```python
from build123d import *

# Parameters (mm, degrees)
SKETCH1_W           = 60
SKETCH1_H           = 28.5
BOSS_EXTRUDE1_DEPTH = 2
SKETCH2_W           = 60
SKETCH2_H           = 2
BOSS_EXTRUDE2_DEPTH = 35
SKETCH3_W           = 41
SKETCH3_H           = 28.5
BOSS_EXTRUDE3_DEPTH = 8
SKETCH4_W           = 20
SKETCH4_H           = 2
BOSS_EXTRUDE4_DEPTH = 20
SKETCH5_W           = 41
SKETCH5_H           = 22
CUT_EXTRUDE1_DEPTH  = 2
SKETCH6_R           = 1.5
CUT_EXTRUDE2_DEPTH  = 2
SKETCH7_R           = 1
BOSS_EXTRUDE5_DEPTH = 5
FILLET1_R           = 10
FILLET2_R           = 10
SKETCH8_R           = 1
CUT_EXTRUDE3_DEPTH  = 2


with BuildPart() as part:
    # Sketch1 → Boss-Extrude1 (new body)
    with BuildSketch(Plane(origin=(0, 0, 0), x_dir=(1, 0, 0), z_dir=(0, 1, 0))):
        Rectangle(SKETCH1_W, SKETCH1_H)
    extrude(amount=BOSS_EXTRUDE1_DEPTH)

    # Sketch2 → Boss-Extrude2 (add)
    with BuildSketch(Plane(origin=(0, 2, 0), x_dir=(1, 0, 0), z_dir=(0, 1, 0))):
        with Locations((0, 13.25)):
            Rectangle(SKETCH2_W, SKETCH2_H)
    extrude(amount=BOSS_EXTRUDE2_DEPTH)

    # Sketch3 → Boss-Extrude3 (add)
    with BuildSketch(Plane(origin=(0, 2, 0), x_dir=(1, 0, 0), z_dir=(0, 1, 0))):
        Rectangle(SKETCH3_W, SKETCH3_H)
    extrude(amount=BOSS_EXTRUDE3_DEPTH)

    # Sketch4 → Boss-Extrude4 (add)
    with BuildSketch(Plane(origin=(0, 10, 0), x_dir=(1, 0, 0), z_dir=(0, 1, 0))):
        with Locations((10.5, -13.25)):
            Rectangle(SKETCH4_W, SKETCH4_H)
    extrude(amount=BOSS_EXTRUDE4_DEPTH)

    # Sketch5 → Cut-Extrude1 (cut)
    with BuildSketch(Plane(origin=(0, 0, -14.25), x_dir=(-1, 0, 0), z_dir=(0, 0, -1))):
        with Locations((0, 21)):
            Rectangle(SKETCH5_W, SKETCH5_H)
    extrude(amount=-CUT_EXTRUDE1_DEPTH, mode=Mode.SUBTRACT)

    # Sketch6 → Cut-Extrude2 (cut)
    with BuildSketch(Plane(origin=(0, 0, -14.25), x_dir=(-1, 0, 0), z_dir=(0, 0, -1))):
        with Locations((-24, 25)):
            Circle(SKETCH6_R)
        with Locations((-24, 15)):
            Circle(SKETCH6_R)
    cut_extrude2 = extrude(amount=-CUT_EXTRUDE2_DEPTH, mode=Mode.SUBTRACT)

    # Mirror1: Cut-Extrude2 across plane
    add(cut_extrude2.mirror(Plane(origin=(0, 0, 0), x_dir=(0, 0, 1), z_dir=(1, 0, 0))), mode=Mode.SUBTRACT)

    # Sketch7 → Boss-Extrude5 (add)
    with BuildSketch(Plane.XY.offset(14.25)):
        with Locations(Location((10.5, 20, 0), (0, 0, 180))):
            Circle(SKETCH7_R)
    extrude(amount=BOSS_EXTRUDE5_DEPTH)

    # Fillet1
    fillet1_edges = [part.edges().sort_by_distance(p)[0] for p in [
        (0.5, 30, 13.25),
        (20.5, 30, 13.25),
    ]]
    fillet(fillet1_edges, radius=FILLET1_R - 0.0001)  # a hair under: the kernel refuses the full size

    # Fillet2
    fillet2_edges = [part.edges().sort_by_distance(p)[0] for p in [
        (-30, 37, -13.25),
        (30, 37, -13.25),
    ]]
    fillet(fillet2_edges, radius=FILLET2_R)

    # Sketch8 → Cut-Extrude3 (cut)
    with BuildSketch(Plane(origin=(0, 2, 0), x_dir=(1, 0, 0), z_dir=(0, 1, 0))):
        with Locations(Location((-26, 0, 0), (0, 0, 270))):
            Circle(SKETCH8_R)
        with Locations(Location((-26, 8, 0), (0, 0, 270))):
            Circle(SKETCH8_R)
        with Locations(Location((-26, -8, 0), (0, 0, 270))):
            Circle(SKETCH8_R)
    cut_extrude3 = extrude(amount=-CUT_EXTRUDE3_DEPTH, mode=Mode.SUBTRACT)

    # Mirror2: Cut-Extrude3 across plane
    add(cut_extrude3.mirror(Plane(origin=(0, 0, 0), x_dir=(0, 0, 1), z_dir=(1, 0, 0))), mode=Mode.SUBTRACT)


solid = part.part
```
The listing builds one solid part. Answer for the finished solid, in the listing's coordinates (mm). A direction names the side the tool comes from. Round coordinates to 2 decimals unless told otherwise and drop trailing zeros. Loops run counter-clockwise (first coordinate to the right, second up) from the corner with the lowest first, then second, coordinate; pieces in that order, holes last. Notation, with made-up numbers: (29.25, -24) -> (86.25, -24) arc R31 cw to (86.25, 5) -> close; hole circle Ø6 at (75, 85). An arc over 180 degrees is marked (long way). Use one line per item in the form item = value.
1. The part is cut by section B-B on x = -4. Determine the outline of the cut face in (y, z), and give its area (3 significant figures).
Answer key:
outline = (0, -14.25) -> (10, -14.25) -> (10, 14.25) -> (0, 14.25) -> close; (32, -14.25) -> (37, -14.25) -> (37, -12.25) -> (32, -12.25) -> close
area = 295 mm²
2. The part is cut by section A-A on z = 0. Determine the outline of the cut face in (x, y), and give its area (3 significant figures).
Answer key:
outline = (-30, 0) -> (-27, 0) -> (-27, 2) -> (-30, 2) -> close; (-25, 0) -> (25, 0) -> (25, 2) -> (20.5, 2) -> (20.5, 10) -> (-20.5, 10) -> (-20.5, 2) -> (-25, 2) -> close; (27, 0) -> (30, 0) -> (30, 2) -> (27, 2) -> close
area = 440 mm²
3. Find the intervals of material crossed by probe 1 along X at (y, z) = (0.45, 8); probe 2 along Y at (x, z) = (-24, -13); probe 3 along Y at (x, z) = (-13.5, 6), in increasing order. Write a range as [from, to].
Answer key:
probe_1 = [-30, -27], [-25, 25], [27, 30]
probe_2 = [0, 13.5], [16.5, 23.5], [26.5, 36.17]
probe_3 = [0, 10]
4. Flat-ended cylindrical pins translate along their axes: pin 1 Ø7.5 at (x, z) = (24.5, 7.5) entering from +Y; pin 2 Ø1 at (y, z) = (12.5, 13.5) entering from -X; pin 3 Ø1.2 at (x, z) = (-26, 8) entering from -Y; pin 4 Ø3 at (y, z) = (9.5, -6) entering from -X. Find the tip coordinate at first contact, or state that the pin passes through.
Answer key:
pin_1 = 2
pin_2 = 0.5
pin_3 = through
pin_4 = -20.5
5. For a pull along Y with two mould halves and no side action, classify faces 6 (the cylindrical face through (-25.5, 15.07, -13.26)), 7 (the flat face through (0, 37, -13)), 8 (the flat face through (11, 20, 19.25)), 9 (the flat face through (-20.5, 21, -13)) as released by +Y, released by -Y, zero draft, split by the parting line, or undercut.
Answer key:
face_6 = undercut
face_7 = released by +Y
face_8 = zero draft
face_9 = undercut
6. The part is cut by section D-D on x = -24. Determine the outline of the cut face in (y, z).
Answer key:
outline = (0, -14.25) -> (13.5, -14.25) -> (13.5, -12.25) -> (2, -12.25) -> (2, 14.25) -> (0, 14.25) -> close; (16.5, -14.25) -> (23.5, -14.25) -> (23.5, -12.25) -> (16.5, -12.25) -> close; (26.5, -14.25) -> (36.17, -14.25) -> (36.17, -12.25) -> (26.5, -12.25) -> close
7. A tool of negligible diameter and unlimited length cuts with its end or side. For faces 1 (the flat face through (10, 20, 12.25)), 2 (the flat face through (0, 6, -14.25)), 3 (the flat face through (0, 32, -13)), 4 (the cylindrical face through (10.717, 20.976, 16.715)), 5 (the cylindrical face through (-27, 1, 0)), from which of +Z, -Z, +X, -X, +Y, -Y can it reach the whole face along a straight path? Write none if from no direction.
Answer key:
face_1 = -Z, +X, -X, +Y
face_2 = -Z, +X, -X, +Y, -Y
face_3 = +Z, -Z
face_4 = +Z
face_5 = +Y, -Y
8. The part is cut by section C-C on y = 6. Determine the outline of the cut face in (x, z), and give its area (3 significant figures).
Answer key:
outline = (-30, -14.25) -> (30, -14.25) -> (30, -12.25) -> (20.5, -12.25) -> (20.5, 14.25) -> (-20.5, 14.25) -> (-20.5, -12.25) -> (-30, -12.25) -> close
area = 1,210 mm²
